Model file for the job. Use its own axes, mm. Face numbers are marked on the shaded views. Give positions to 0.01 mm unless a question says otherwise; leave off trailing zeros. Loops run counter-clockwise (first coordinate to the right, second up) from the corner with the lowest first, then second, coordinate; pieces in that order, holes last. Notation, with made-up numbers: M -7.5,36.5 L 33.5,36.5 A16 cw 33.5,58.5 Z; hole C -9,13 d8. An arc over 180 degrees is marked long. Answer in a Markdown table with one row per item.
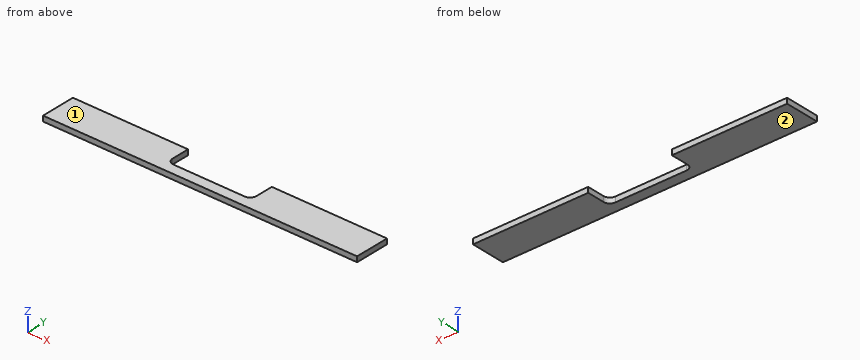
```python
from build123d import *

# Parameters (mm, degrees)
F0_W     = 1500
F0_H     = 165
F1_DEPTH = 25
F3_DEPTH = 25


with BuildPart() as f1:
    # F0 (on Top) → F1 (new body)
    with BuildSketch(Plane.XY):
        Rectangle(F0_W, F0_H)
    extrude(amount=F1_DEPTH)

    # F2 (on face) → F3 (cut, through all)
    with BuildSketch(Plane.XY.offset(25)):
        with BuildLine():
            Line((200, 82.5), (-200, 82.5))
            Line((-200, 82.5), (-200, -2.5))
            ThreePointArc((-200, -2.5), (-191.213203, -23.713203), (-170, -32.5))
            Line((-170, -32.5), (0, -32.5))
            Line((0, -32.5), (170, -32.5))
            ThreePointArc((170, -32.5), (191.213203, -23.713203), (200, -2.5))
            Line((200, -2.5), (200, 82.5))
        make_face()
    extrude(amount=-F3_DEPTH, mode=Mode.SUBTRACT)


solid = f1.part
```
Q1. Probe probe 1 along X at (y, z) = (69.5, 8); probe 2 along X at (y, z) = (-4.5, 17.25); probe 3 along Y at (x, z) = (-121.5, 5). List the from-to ranges inside material, lowest first.
Reported:
| item | result |
|---|---|
| probe 1 | -750 to -200, 200 to 750 |
| probe 2 | -750 to -199.93, 199.93 to 750 |
| probe 3 | -82.5 to -32.5 |
Q2. Saw through at A-A (y = 24). Give the cut face in (x, z).
Reported:
| item | result |
|---|---|
| outline | M -750,0 L -200,0 L -200,25 L -750,25 Z; M 200,0 L 750,0 L 750,25 L 200,25 Z |
Q3. Mould opens along Z. For the marked faces 1 and 2 say: released by +Z, released by -Z, zero draft, split by the parting line, or undercut.
Reported:
| item | result |
|---|---|
| face 1 | released by +Z |
| face 2 | released by -Z |
Q4. Saw through at B-B (z = 15.5). Give the cut face in (x, y), and give its area (3 significant figures).
Reported:
| item | result |
|---|---|
| outline | M -750,-82.5 L 750,-82.5 L 750,82.5 L 200,82.5 L 200,-2.5 A30 cw 170,-32.5 L -170,-32.5 A30 cw -200,-2.5 L -200,82.5 L -750,82.5 Z |
| area | 202,000 mm² |
Q5. Drop flat-ended pins along their axis: pin 1 (1 mm diameter, centred on x = -311, y = -9, fed in from -Z); pin 2 (12 mm diameter, centred on x = -81, z = 18.5, fed in from +Y). Give the stop position or say it passes through.
Reported:
| item | result |
|---|---|
| pin 1 | z = 0 |
| pin 2 | y = -32.5 |
